Can you work these out from the drawing? Everything is in mm from the part's minimum corner. A direction names the side the tool comes from. Coordinates: 2 decimals unless noted, no trailing zeros. Order: outer loops, then holes, each group sorted by start corner. A loop starts at its lowest first (then second) coordinate and runs counter-clockwise, first axis right, second up. Notation, with made-up numbers: (37.5, 1.25) - (66.5, 1.25) arc R21 ccw to (66.5, 36.25) - close; hole circle Ø4 at (-2.75, 0). An arc over 180 degrees is marked (long way). Answer as CSV lines item,"result". Start each with the question number.
Q1. Suppose I cut it at A-A (z = 17). Please give me the cut outline in (x, y) (1 decimal).
Q2. For the marked faces 1 and 2, which set-ups out of +Z, -Z, +X, -X, +Y, -Y let a thin tool reach every point of the face, with its end or its side?
Q3. Suppose I cut it at C-C (x = 67). Please give me the cut outline in (y, z) (1 decimal), then the cut area to 3 significant figures.
Q4. I need wall thicknesses on line 1 (X direction, y = 26, z = 3) (1 decimal); line 2 (Z direction, x = 64, y = 67) (1 decimal); line 3 (X direction, y = 57, z = 18.75) (1 decimal). Which ranges of each line are inside material? Lowest first, please.
Q5. Suppose I cut it at D-D (y = 8). Please give me the cut outline in (x, z) (1 decimal).
Q6. Thinking about a two-plate mould opening in Y: for the marked faces 3 and 4, which applies, released by +Y, released by -Y, zero draft, split by the parting line, or undercut?
Q7. Suppose I cut it at B-B (y = 41). Please give me the cut outline in (x, z) (1 decimal), then the cut area to 3 significant figures.
Q8. For pin 1 Ø0.6 at (x, z) = (52.5, 3) entering from -Y; pin 2 Ø10 at (y, z) = (36.5, 19) entering from +X (1 decimal); pin 3 Ø5 at (x, z) = (37, 13.5) entering from -Y; pin 4 Ø1.9 at (x, z) = (39.5, 9) entering from +Y, each with a flat end and sliding along its axis, tell me the tip position at first contact or that it passes through.
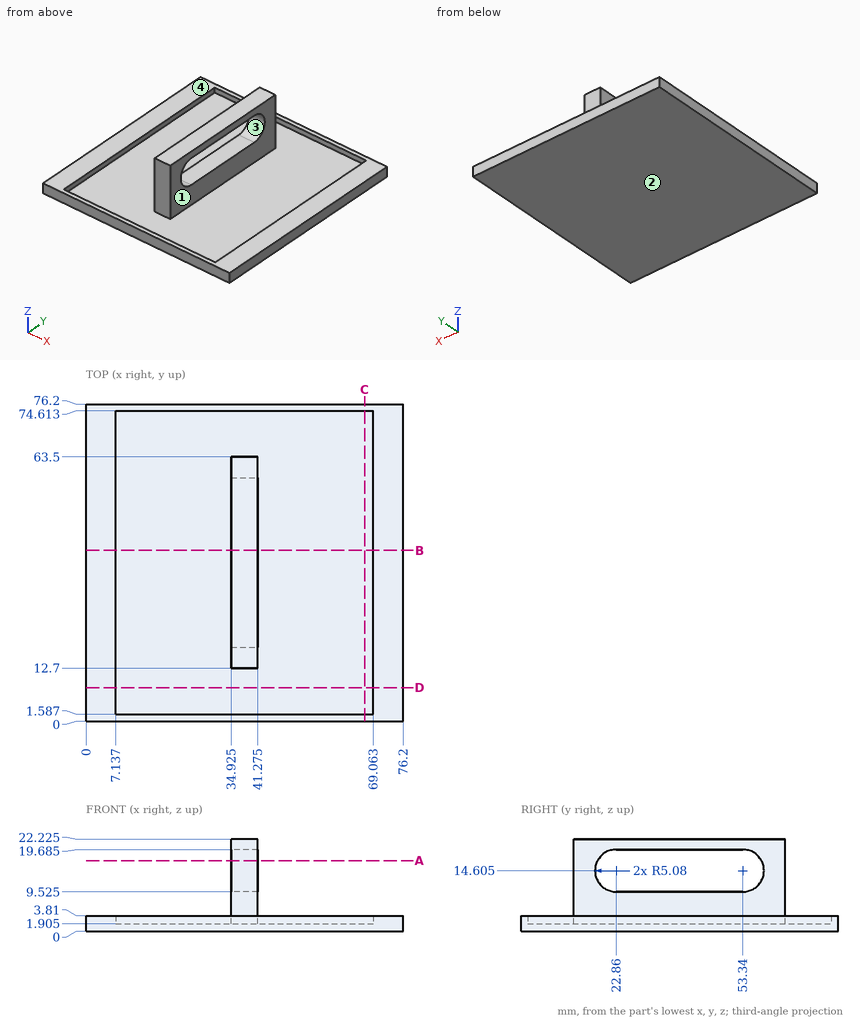
Here are the results:
1,outline,"(34.9, 12.7) - (41.3, 12.7) - (41.3, 18.4) - (34.9, 18.4) - close; (34.9, 57.8) - (41.3, 57.8) - (41.3, 63.5) - (34.9, 63.5) - close"
2,face 1,"+Z"
2,face 2,"-Z, +X, -X, +Y, -Y"
3,outline,"(0, 0) - (76.2, 0) - (76.2, 3.8) - (74.6, 3.8) - (74.6, 1.9) - (1.6, 1.9) - (1.6, 3.8) - (0, 3.8) - close"
3,area,"151 mm²"
4,line 1,"x = 0 to 7.1, 34.9 to 41.3, 69.1 to 76.2"
4,line 2,"z = 0 to 1.9"
4,line 3,"x = 34.9 to 41.3"
5,outline,"(0, 0) - (76.2, 0) - (76.2, 3.8) - (69.1, 3.8) - (69.1, 1.9) - (7.1, 1.9) - (7.1, 3.8) - (0, 3.8) - close"
6,face 3,"undercut"
6,face 4,"zero draft"
7,outline,"(0, 0) - (76.2, 0) - (76.2, 3.8) - (69.1, 3.8) - (69.1, 1.9) - (41.3, 1.9) - (41.3, 9.5) - (34.9, 9.5) - (34.9, 1.9) - (7.1, 1.9) - (7.1, 3.8) - (0, 3.8) - close; (34.9, 19.7) - (41.3, 19.7) - (41.3, 22.2) - (34.9, 22.2) - close"
7,area,"237 mm²"
8,pin 1,"stops at y = 0"
8,pin 2,"stops at x = 41.3"
8,pin 3,"stops at y = 12.7"
8,pin 4,"stops at y = 63.5"
